Design review of the part built by this model. Coordinates are the model's own, in mm. A direction names the side the tool comes from. Give positions to 0.01 mm unless a question says otherwise; leave off trailing zeros. Loops run counter-clockwise (first coordinate to the right, second up) from the corner with the lowest first, then second, coordinate; pieces in that order, holes last. Notation, with made-up numbers: (81.5, -12.5) - (105.5, -12.5) arc R16 cw to (105.5, -2.5) - close; hole circle Ø1 at (-16, 21). An arc over 180 degrees is marked (long way). Write each question's results on one line, items separated by ' | '.
from build123d import *

# Parameters (mm, degrees)
SKETCH1_R           = 7.5
BOSS_EXTRUDE1_DEPTH = 220
FILLET1_R           = 2
BOSS_EXTRUDE2_REACH = 259.5
SKETCH3_W           = 4.49
SKETCH3_H           = 6.99


with BuildPart() as part:
    # Sketch1 → Boss-Extrude1 (new body)
    with BuildSketch(Plane.XY):
        Circle(SKETCH1_R)
    extrude(amount=BOSS_EXTRUDE1_DEPTH)

    # Fillet1
    fillet1_edges = [part.edges().sort_by_distance(p)[0] for p in [
        (-7.5, 0, 0),
        (-7.5, 0, 220),
    ]]
    fillet(fillet1_edges, radius=FILLET1_R)

    # Sketch3 → Boss-Extrude2 (add, up to next)
    with BuildSketch(Plane(origin=(0, 250, 0), x_dir=(1, 0, 0), z_dir=(0, 1, 0)), mode=Mode.PRIVATE) as boss_extrude2_sk1:
        with Locations((0, -110)):
            Rectangle(SKETCH3_W, SKETCH3_H)
    boss_extrude2_tool1 = extrude(boss_extrude2_sk1.sketch, amount=-BOSS_EXTRUDE2_REACH, mode=Mode.PRIVATE) - part.part
    add(boss_extrude2_tool1.solids().sort_by_distance((0, 250, 110))[0])


solid = part.part
(1) Take a section at A-A on y = 129.5. Give the boundary of the cut face in (x, z) (3 decimals), plus the area to 3 significant figures.
Answers below:
outline: (-2.245, 106.505) - (2.245, 106.505) - (2.245, 113.495) - (-2.245, 113.495) - close | area: 31.4 mm2
(2) Insertion check: P1, Ø5.5, axis at y = 70, z = 108.5, coming from the -X side (3 decimals); P2, Ø1.3, axis at x = -0.5, y = 96, coming from the -Z side (3 decimals); P3, Ø6, axis at x = 5.5, z = 130, coming from the +Y side; P4, Ø3, axis at x = 4.5, y = 201.5, coming from the -Z side. Each pin has a flat end and moves straight along its axis. Give the tip position at first contact, or say it passes through.
Answers below:
P1: x = -2.245 | P2: z = 106.505 | P3: y = 7.07 | P4: through
(3) Wall thickness on line 1 along Y through (x, z) = (0.75, 128); line 2 along Z through (x, y) = (-0.5, 136) (3 decimals); line 3 along Y through (x, z) = (1, 142): over which ranges is each line inside the solid? List them lowest first. Write a range as from..to.
Answers below:
line 1: -7.46..7.46 | line 2: 106.505..113.495 | line 3: -7.43..7.43
(4) Take a section at B-B on z = 182. Give the boundary of the cut face in (x, y).
Answers below:
outline: circle Ø15 at (0, 0)
(5) Tool access review of faces 1 (the flat face through (2.245, 130, 110)), 2 (the flat face through (0, 0, 220)), 3 (the flat face through (-2.245, 130, 110)): name each direction out of +Z, -Z, +X, -X, +Y, -Y from which nothing blocks a thin tool from reaching the whole face with its end or side.
Answers below:
face 1: +Z, -Z, +X, +Y | face 2: +Z, +X, -X, +Y, -Y | face 3: +Z, -Z, -X, +Y
